CAD build for the part. Positions are in the model's coordinates, mm. Face numbers are marked on the shaded views. A direction names the side the tool comes from. Round coordinates to 2 decimals unless told otherwise and drop trailing zeros. Order: outer loops, then holes, each group sorted by start corner. A loop starts at its lowest first (then second) coordinate and runs counter-clockwise, first axis right, second up. Notation, with made-up numbers: (-14.5, 42) -> (14.5, 42) arc R19 ccw to (14.5, 50) -> close; hole circle Ø11 at (-29, 83.5). An arc over 180 degrees is marked (long way). Answer as CSV lines item,"result". Start each with the question number.
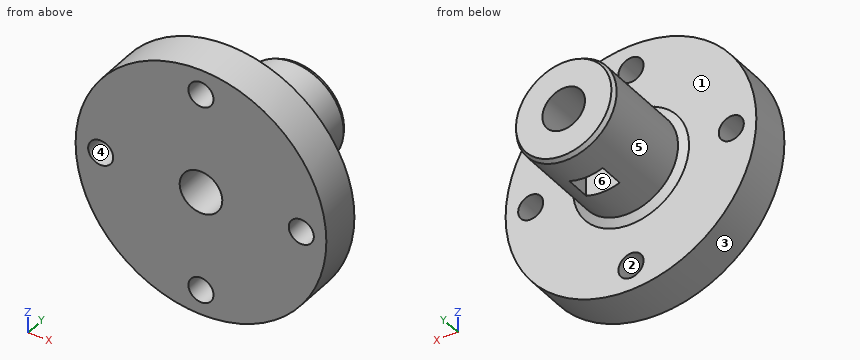
from build123d import *

# Parameters (mm, degrees)
SKETCH_1_R          = 15
EXTRUDE_1_DEPTH     = 5
SKETCH_4_R          = 6
EXTRUDE_2_DEPTH     = 12
SKETCH_5_R          = 2.55
CUT_EXTRUDE_1_DEPTH = 28.184554438
SKETCH_6_W          = 4
SKETCH_6_H          = 3
CUT_EXTRUDE_2_DEPTH = 28.184554438
CHAMFER_1_SIZE      = 0.947
CHAMFER_1_SIZE2     = 0.546750705
CHAMFER_2_SIZE      = 0.5
CHAMFER_2_SIZE2     = 0.288675135
SKETCH_7_R          = 1.5
CUT_EXTRUDE_3_DEPTH = 25.372115214


with BuildPart() as part:
    # 草图1 → 凸台-拉伸1 (new body)
    with BuildSketch(Plane(origin=(0, 0, 0), x_dir=(1, 0, 0), z_dir=(0, 1, 0))):
        with Locations(Location((0, 0, 0), (0, 0, 270))):
            Circle(SKETCH_1_R)
    extrude(amount=EXTRUDE_1_DEPTH)

    # 草图4 → 凸台-拉伸2 (add)
    with BuildSketch(Plane(origin=(0, 5, 0), x_dir=(1, 0, 0), z_dir=(0, 1, 0))):
        with Locations(Location((0, 0, 0), (0, 0, 270))):
            Circle(SKETCH_4_R)
    extrude(amount=EXTRUDE_2_DEPTH)

    # 草图5 → 切除-拉伸1 (cut, through all)
    with BuildSketch(Plane(origin=(0, 17, 0), x_dir=(1, 0, 0), z_dir=(0, 1, 0))):
        with Locations(Location((0, 0, 0), (0, 0, 270))):
            Circle(SKETCH_5_R)
    extrude(amount=-CUT_EXTRUDE_1_DEPTH, mode=Mode.SUBTRACT)

    # 草图6 → 切除-拉伸2 (cut, through all)
    with BuildSketch(Plane.XY):
        with Locations((0, 11.5)):
            Rectangle(SKETCH_6_W, SKETCH_6_H)
    extrude(amount=-CUT_EXTRUDE_2_DEPTH, mode=Mode.SUBTRACT)

    # 倒角1
    chamfer_1_edges = [part.edges().sort_by_distance(p)[0] for p in [
        (0, 5, -6),
    ]]
    chamfer_1_side = [part.faces().sort_by_distance(p)[0] for p in [
        (0, 5, -14.575735931),
    ]]
    chamfer(chamfer_1_edges, length=CHAMFER_1_SIZE, length2=CHAMFER_1_SIZE2, reference=chamfer_1_side[0])

    # 倒角2
    chamfer_2_edges = [part.edges().sort_by_distance(p)[0] for p in [
        (0, 17, -6),
    ]]
    chamfer_2_side = [part.faces().sort_by_distance(p)[0] for p in [
        (0, 11.273375352, -6),
    ]]
    chamfer(chamfer_2_edges, length=CHAMFER_2_SIZE, length2=CHAMFER_2_SIZE2, reference=chamfer_2_side[0])

    # 草图7 → 切除-拉伸3 (cut, through all)
    with BuildSketch(Plane(origin=(0, 5, 0), x_dir=(1, 0, 0), z_dir=(0, 1, 0))):
        with Locations(Location((0, 12, 0), (0, 0, 270))):
            Circle(SKETCH_7_R)
        with Locations(Location((-12, 0, 0), (0, 0, 270))):
            Circle(SKETCH_7_R)
        with Locations(Location((12, 0, 0), (0, 0, 270))):
            Circle(SKETCH_7_R)
        with Locations(Location((0, -12, 0), (0, 0, 270))):
            Circle(SKETCH_7_R)
    extrude(amount=-CUT_EXTRUDE_3_DEPTH, mode=Mode.SUBTRACT)


solid = part.part
Item 1: Band-saw the part on B-B, the plane x = 0. Give the cut face in (y, z), and give its area (3 significant figures).
Item 2: Mould opens along X. For the marked faces 1, 2 and 3 say: released by +X, released by -X, zero draft, split by the parting line, or undercut.
Item 3: Band-saw the part on A-A, the plane z = -12. Give the cut face in (x, y), and give its area (3 significant figures).
Item 4: Probe line 1 (X direction, y = 2.1, z = 0); line 2 (Y direction, x = -10, z = 3.75); line 3 (X direction, y = 13.5, z = 1.75). List the from-to ranges inside material, lowest first.
Item 5: Pin check, flat tips, straight feed: pin 1 (5 mm diameter, centred on x = 0, z = -12, fed in from +Y); pin 2 (6 mm diameter, centred on y = 2, z = 11.5, fed in from -X); pin 3 (4 mm diameter, centred on x = 0, z = 0, fed in from -Y); pin 4 (2.5 mm diameter, centred on y = 11, z = -3.5, fed in from -X). Stop position of each tip, or through.
Item 6: Band-saw the part on D-D, the plane y = 14.25. Give the cut face in (x, z).
Item 7: Tool access for the marked faces 4, 5 and 6: list every direction of +Z, -Z, +X, -X, +Y, -Y with a clear straight run to the whole face (end or side of a thin tool).
Item 8: Band-saw the part on C-C, the plane x = 12. Give the cut face in (y, z).
Values:
1,outline,"(0, -15) -> (5, -15) -> (5, -13.5) -> (0, -13.5) -> close; (0, -10.5) -> (5, -10.5) -> (5, -6.95) -> (5.55, -6) -> (10, -6) -> (10, -2.55) -> (0, -2.55) -> close; (0, 2.55) -> (17, 2.55) -> (17, 5.71) -> (16.5, 6) -> (5.55, 6) -> (5, 6.95) -> (5, 10.5) -> (0, 10.5) -> close; (0, 13.5) -> (5, 13.5) -> (5, 15) -> (0, 15) -> close; (13, -6) -> (16.5, -6) -> (17, -5.71) -> (17, -2.55) -> (13, -2.55) -> close"
1,area,"167 mm²"
2,face 1,"zero draft"
2,face 2,"undercut"
2,face 3,"split by the parting line"
3,outline,"(-9, 0) -> (-1.5, 0) -> (-1.5, 5) -> (-9, 5) -> close; (1.5, 0) -> (9, 0) -> (9, 5) -> (1.5, 5) -> close"
3,area,"75.0 mm²"
4,line 1,"-15 to -13.5, -10.5 to -2.55, 2.55 to 10.5, 13.5 to 15"
4,line 2,"0 to 5"
4,line 3,"-5.74 to -1.85, 1.85 to 5.74"
5,pin 1,"y = 5"
5,pin 2,"x = -12.36"
5,pin 3,"through"
5,pin 4,"x = -5.56"
6,outline,"circle Ø12 at (0, 0); hole circle Ø5.1 at (0, 0)"
7,face 4,"+Y, -Y"
7,face 5,"+Y"
7,face 6,"-Z"
8,outline,"(0, -9) -> (5, -9) -> (5, -1.5) -> (0, -1.5) -> close; (0, 1.5) -> (5, 1.5) -> (5, 9) -> (0, 9) -> close"
